Build history of the part. All positions in model axes, mm. A direction names the side the tool comes from. Give positions to 0.01 mm unless a question says otherwise; leave off trailing zeros. Loops run counter-clockwise (first coordinate to the right, second up) from the corner with the lowest first, then second, coordinate; pieces in that order, holes last.
1) Band-saw the part on B-B on x = 14. List the corners of the cut face in (y, z), then the cut area to 3 significant figures.
2) Two-plate mould, pull along Y, no slides. Class faces 4 (the flat face through (-5, -46.586, 2)), 5 (the cylindrical face through (13.51, 85.19, 1.58)), 6 (the flat face through (-12.825, -48, 2)): +Y half, -Y half, draft (parallel to the pull), parting line (faces both ways), or undercut.
3) Flat gauge pins, fed straight in: P1, Ø1, axis at x = 15.5, z = 2, coming from the -Y side; P2, Ø1.6, axis at y = -49, z = 1.5, coming from the -X side; P3, Ø1.6, axis at y = -48, z = 2.5, coming from the +X side. Where does each tip first touch, or does it go through?
4) Wall check: line 1 (Y direction, x = 12.5, z = 1.75); line 2 (Y direction, x = 26, z = 0.25); line 3 (X direction, y = 30, z = 1). Give the ranges that are in metal, low to high.
5) Band-saw the part on A-A on z = 1. List the corners of the cut face in (x, y), then the cut area to 3 significant figures.
6) 3-axis set-ups, long thin cutter, end or side, ignore diameter. For faces 1 (the flat face through (25, -46.586, 2)), 2 (the flat face through (10, 26, 3.2)), 3 (the flat face through (-25, -46.586, 2)): which of +Z, -Z, +X, -X, +Y, -Y reach the whole face in a straight line?
7) Band-saw the part on C-C on y = 4.5. List the corners of the cut face in (x, z).
8) Band-saw the part on D-D on x = 24.5. List the corners of the cut face in (y, z), then the cut area to 3 significant figures.
```python
from build123d import *

# Parameters (mm, degrees)
F0_R     = 2.5
F1_DEPTH = 3.2


with BuildPart() as f1:
    # F0 (on Top) → F1 (new body)
    with BuildSketch(Plane.XY):
        Polygon((34.059358, 100.213571), (-1.940642, 100.213571), (-27.825443, -46.586429), (-22.825443, -46.586429), (-22.825443, -49.786429), (-17.825443, -49.786429), (-17.825443, -46.586429), (-12.825443, -46.586429), (-12.825443, -49.786429), (-7.825443, -49.786429), (-7.825443, -46.586429), (-2.825443, -46.586429), (-2.825443, -49.786429), (2.174557, -49.786429), (2.174557, -46.586429), (7.174557, -46.586429), (7.174557, -49.786429), (12.174557, -49.786429), (12.174557, -46.586429), (17.174557, -46.586429), (17.174557, -49.786429), (22.174557, -49.786429), (22.174557, -46.586429), (27.174557, -46.586429), (27.174557, -49.786429), (32.174557, -49.786429), align=None)
        with Locations((-7.825443, -14.086429)):
            Circle(F0_R, mode=Mode.SUBTRACT)
        with Locations((13.837886, 82.713571)):
            Circle(F0_R, mode=Mode.SUBTRACT)
    extrude(amount=F1_DEPTH)


solid = f1.part
```
Findings below:
1. outline: (-46.59, 0) - (80.22, 0) - (80.22, 3.2) - (-46.59, 3.2) - close; (85.21, 0) - (100.21, 0) - (100.21, 3.2) - (85.21, 3.2) - close
1. area: 454 mm2
2. face 4: -Y half
2. face 5: undercut
2. face 6: draft
3. P1: stops at y = -46.59
3. P2: stops at x = -22.83
3. P3: stops at x = 32.21
4. line 1: y = -46.59 to 80.6, 84.83 to 100.21
4. line 2: y = -46.59 to 100.21
4. line 3: x = -14.32 to 33.18
5. outline: (-27.83, -46.59) - (-22.83, -46.59) - (-22.83, -49.79) - (-17.83, -49.79) - (-17.83, -46.59) - (-12.83, -46.59) - (-12.83, -49.79) - (-7.83, -49.79) - (-7.83, -46.59) - (-2.83, -46.59) - (-2.83, -49.79) - (2.17, -49.79) - (2.17, -46.59) - (7.17, -46.59) - (7.17, -49.79) - (12.17, -49.79) - (12.17, -46.59) - (17.17, -46.59) - (17.17, -49.79) - (22.17, -49.79) - (22.17, -46.59) - (27.17, -46.59) - (27.17, -49.79) - (32.17, -49.79) - (34.06, 100.21) - (-1.94, 100.21) - close; hole circle Ø5 at (-7.83, -14.09); hole circle Ø5 at (13.84, 82.71)
5. area: 7,110 mm2
6. face 1: +Z, -Z, -Y
6. face 2: +Z, +X, -X, +Y, -Y
6. face 3: +Z, -Z, -X, -Y
7. outline: (-18.82, 0) - (32.86, 0) - (32.86, 3.2) - (-18.82, 3.2) - close
8. outline: (-46.59, 0) - (100.21, 0) - (100.21, 3.2) - (-46.59, 3.2) - close
8. area: 470 mm2
